For this review, take the finished solid that the model builds, in its own axes (mm). A direction names the side the tool comes from. Give positions to 0.01 mm unless a question says otherwise; leave off trailing zeros. Write each loop counter-clockwise with the first axis right and the second up, starting at its lowest first coordinate (ties: lowest second). Pieces come first, ordered by that corner, then holes. Notation, with made-up numbers: M 31.5,-33.75 L 70.5,-33.75 A15 ccw 70.5,-15.75 Z; hole C 35,49.25 d2. An arc over 180 degrees is marked long. Answer as a JSON object with one key per item and string values. Group by question number.
Autodesk Inventor part; units mm, degrees
ref_plane "YZ Plane" through (0, 0, 0) normal (1, 0, 0) x (0, 1, 0)
ref_plane "XZ Plane" through (0, 0, 0) normal (0, 1, 0) x (-1, 0, 0)
ref_plane "XY Plane" through (0, 0, 0) normal (0, 0, 1) x (1, 0, 0)
sketch "Sketch1" plane through (0, 0, 0) normal (0, 1, 0) x (-1, 0, 0)
  line L0 (0, 0) -> (42.3, 0)
  line L1 (42.3, 0) -> (42.3, 42.3)
  line L2 (42.3, 42.3) -> (0, 42.3)
  line L3 (0, 42.3) -> (0, 0)
  dimension "d0" = 42.3
  dimension "d1" = 42.3
extrude "Extrusion1" add sketch "Sketch1" along normal blind 60
sketch "Sketch2" plane through (0, 60, 0) normal (0, 1, 0) x (1, 0, 0)
  line L0 (0, 0) -> (-42.3, 0)
  line L1 (0, -42.3) -> (0, 0)
  circle A0 centre (-21.15, -21.15) radius 11
  point P0 (0, -2)
  point P1 (-2, 0)
  point P2 (-40.3, 0)
  point P3 (0, -40.3)
  dimension "d6" = 22
  dimension "d7" = 21.15
  dimension "d8" = 21.15
extrude "Extrusion2" add sketch "Sketch2" along normal blind 2
sketch "Sketch3" plane through (-21.15, 62, 21.15) normal (0, 1, 0) x (1, 0, 0)
  circle A0 centre (0, 0) radius 11
  circle A1 centre (0, 0) radius 2.5
  point P0 (21.15, 21.15)
  dimension "d11" = 5
extrude "Extrusion3" add sketch "Sketch3" along normal blind 22 contours A1
sketch "Sketch4" plane through (-21.15, 84, 21.15) normal (0, 1, 0) x (1, 0, 0)
  circle A0 centre (0, 0) radius 2.5
  line L0 (-1.5, 2) -> (1.5, 2)
  point P0 (21.15, 21.15)
  dimension "d14" = 2
extrude "Extrusion4" cut sketch "Sketch4" against normal blind 21 contours L0 A0 picked at (-0.3466, 2.0912)
sketch "Sketch5" plane through (0, 60, 0) normal (0, 1, 0) x (1, 0, 0)
  line L0 (-42.3, 0) -> (-42.3, -42.3)
  line L1 (-42.3, -42.3) -> (0, -42.3)
  circle A0 centre (-36.65, -5.65) radius 1.5
  circle A1 centre (-5.65, -5.65) radius 1.5
  circle A2 centre (-5.65, -36.65) radius 1.5
  circle A3 centre (-36.65, -36.65) radius 1.5
  point P0 (-42.3, -2)
  point P1 (-42.3, -40.3)
  point P2 (-40.3, -42.3)
  point P3 (-2, -42.3)
  point P4 (0, 0)
  dimension "d17" = 3
  dimension "d18" = 3
  dimension "d19" = 3
  dimension "d20" = 3
  dimension "d21" = 31
  dimension "d22" = 5.65
  dimension "d23" = 31
  dimension "d24" = 5.65
extrude "Extrusion5" cut sketch "Sketch5" against normal blind 4.5
chamfer "Chamfer1" distance 4 angle 45 4 edges at (-42.3, 30, 0) (-42.3, 30, 42.3) (0, 30, 0) (0, 30, 42.3)
properties part number "StepperMotorNema17"
Item 1: Draft analysis for pull direction Z (two halves, no side actions). For faces 1 (the flat face through (-2, 29.6, 40.3)), 2 (the flat face through (-21, 0, 21)), 3 (the cylindrical face through (-38.15, 57.78, 5.58)), state which applies: released by +Z, released by -Z, zero draft, split by the parting line, or undercut.
Item 2: Consider section D-D (z = 11.5). Give the boundary of the cut face in (x, y).
Item 3: Consider section B-B (z = 21.15). Give the boundary of the cut face in (x, y), plus the area to 3 significant figures.
Item 4: Consider section C-C (x = -5.65). Give the boundary of the cut face in (y, z), plus the area to 3 significant figures.
Item 5: Machinability: for faces 4 (the cylindrical face through (-29.26, 60.99, 28.58)), 5 (the flat face through (-21, 74, 19.15)), 6 (the flat face through (-40.3, 30.4, 2)), which of the approach directions +Z, -Z, +X, -X, +Y, -Y give a long, thin tool a straight path to every point of the face, cutting with its end or side? Answer none if there is none.
Item 6: Insertion check: P1, Ø2.5, axis at x = -5, z = 5, coming from the +Y side; P2, Ø1.8, axis at x = -5.65, z = 36.65, coming from the +Y side; P3, Ø2.5, axis at x = -21, y = 78, coming from the -Z side. Each pin has a flat end and moves straight along its axis. Give the tip position at first contact, or say it passes through.
Item 7: To check wall thickness, follow probe 1 along X at (y, z) = (58.05, 36.65); probe 2 along Z at (x, y) = (-36.65, 58.85); probe 3 along X at (y, z) = (58, 5). State the ranges of each line that lie inside material, in increasing order.
Item 8: Consider section A-A (y = 35.5). Give the boundary of the cut face in (x, z), plus the area to 3 significant figures.
Result set:
{
 "1": {"face 1": "released by +Z", "face 2": "zero draft", "face 3": "undercut"},
 "2": {"outline": "M -42.3,0 L 0,0 L 0,60 L -15.87,60 L -15.87,62 L -26.43,62 L -26.43,60 L -42.3,60 Z"},
 "3": {"outline": "M -42.3,0 L 0,0 L 0,60 L -10.15,60 L -10.15,62 L -18.65,62 L -18.65,84 L -23.65,84 L -23.65,62 L -32.15,62 L -32.15,60 L -42.3,60 Z", "area": "2,690 mm^2"},
 "4": {"outline": "M 0,0 L 60,0 L 60,4.15 L 55.5,4.15 L 55.5,7.15 L 60,7.15 L 60,35.15 L 55.5,35.15 L 55.5,38.15 L 60,38.15 L 60,42.3 L 0,42.3 Z", "area": "2,510 mm^2"},
 "5": {"face 4": "+Y", "face 5": "-Z, +X, -X, +Y", "face 6": "-Z, -X, +Y, -Y"},
 "6": {"P1": "stops at y = 60", "P2": "stops at y = 55.5", "P3": "stops at z = 19.15"},
 "7": {"probe 1": "x = -42.3 to -38.15, -35.15 to -7.15, -4.15 to 0", "probe 2": "z = 0 to 4.15, 7.15 to 35.15, 38.15 to 42.3", "probe 3": "x = -42.3 to -38, -35.3 to -7, -4.3 to 0"},
 "8": {"outline": "M -42.3,4 L -38.3,0 L -4,0 L 0,4 L 0,38.3 L -4,42.3 L -38.3,42.3 L -42.3,38.3 Z", "area": "1,760 mm^2"}
}
